Can you work these out from the model? Positions are in its coordinate system, mm. Face numbers are marked on the shaded views. A direction names the side the tool comes from. Coordinates: 2 decimals unless noted, no trailing zeros. Loops run counter-clockwise (first coordinate to the right, second up) from the corner with the lowest first, then second, coordinate; pieces in that order, holes last. Notation, with made-up numbers: (13.25, 9) -> (55.25, 9) arc R29 cw to (55.25, 31) -> close; hole circle Ø11 at (-8.5, 20.5). An arc over 180 degrees is marked (long way). Put each result on its own line as item: value. Start each with the question number.
Item 1: For the marked faces 1, 2, 3 and 4, which set-ups out of +Z, -Z, +X, -X, +Y, -Y let a thin tool reach every point of the face, with its end or its side?
Item 2: We'd pull the mould along Z, two halves only. Please class the marked faces 5, 6, 7 and 8: pulls with the +Z half, pulls with the -Z half, needs draft (parallel to the pull), parting line crosses it, or undercut.
Item 3: If we section it at A-A on z = -65.5: Please give me the cut outline in (x, y), plus the area to 3 significant figures.
Item 4: If we section it at C-C on y = 19: Please give me the cut outline in (x, z).
Item 5: If we section it at B-B on x = 30.5: Please give me the cut outline in (y, z), plus the area to 3 significant figures.
Item 6: Please list where these lines run through material, in increasing order: L1, parallel to Z at x = -146, y = 3; L2, parallel to X at y = 8.5, z = 21; L3, parallel to X at y = 27, z = -20. Write a range as from..to.
Item 7: Will these pins go through, and if not, where does the flat tip stop? P1, Ø4, axis at x = -62, z = 29, coming from the +Y side; P2, Ø1, axis at y = 29, z = -21, coming from the +X side; P3, Ø5, axis at y = 42.5, z = 27.5, coming from the -X side.
```python
from build123d import *

# Parameters (mm, degrees)
SKETCH1_W           = 300
SKETCH1_H           = 200
SKETCH1_R           = 2
BOSS_EXTRUDE1_DEPTH = 5
CUT_EXTRUDE1_REACH  = 182.347
SKETCH3_W           = 80
SKETCH3_H           = 180
SKETCH4_W           = 30
SKETCH4_H           = 60
BOSS_EXTRUDE2_DEPTH = 50
BOSS_EXTRUDE3_DEPTH = 45
SKETCH7_R           = 1.5
CUT_EXTRUDE2_DEPTH  = 5


with BuildPart() as part:
    # Sketch1 → Boss-Extrude1 (new body)
    with BuildSketch(Plane(origin=(0, 0, 0), x_dir=(1, 0, 0), z_dir=(0, 1, 0))):
        Rectangle(SKETCH1_W, SKETCH1_H)
        with Locations(Location((-146, 96, 0), (0, 0, 270))):
            Circle(SKETCH1_R, mode=Mode.SUBTRACT)
        with Locations(Location((146, 96, 0), (0, 0, 90))):
            Circle(SKETCH1_R, mode=Mode.SUBTRACT)
        with Locations(Location((146, -96, 0), (0, 0, 270))):
            Circle(SKETCH1_R, mode=Mode.SUBTRACT)
        with Locations(Location((-146, -96, 0), (0, 0, 90))):
            Circle(SKETCH1_R, mode=Mode.SUBTRACT)
    extrude(amount=BOSS_EXTRUDE1_DEPTH)

    # Sketch3 → Cut-Extrude1 (cut, up to next)
    with BuildSketch(Plane(origin=(0, 5, 0), x_dir=(1, 0, 0), z_dir=(0, 1, 0)), mode=Mode.PRIVATE) as cut_extrude1_sk1:
        Rectangle(SKETCH3_W, SKETCH3_H)
    cut_extrude1_tool1 = extrude(cut_extrude1_sk1.sketch, amount=-CUT_EXTRUDE1_REACH, mode=Mode.PRIVATE) & part.part
    add(cut_extrude1_tool1.solids().sort_by_distance((0, 5, 0))[0], mode=Mode.SUBTRACT)

    # Sketch4 → Boss-Extrude2 (add)
    with BuildSketch(Plane(origin=(0, 5, 0), x_dir=(1, 0, 0), z_dir=(0, 1, 0))):
        with Locations((-100, 0)):
            Rectangle(SKETCH4_W, SKETCH4_H)
    boss_extrude2 = extrude(amount=BOSS_EXTRUDE2_DEPTH)

    # Sketch5 → Boss-Extrude3 (add)
    with BuildSketch(Plane(origin=(-85, 0, 0), x_dir=(0, 0, -1), z_dir=(1, 0, 0))):
        with BuildLine():
            Line((-26.2, 38.191891423), (-30, 38.191891423))
            Line((-30, 38.191891423), (-30, 5))
            Line((-30, 5), (30, 5))
            Line((30, 5), (30, 38.191891423))
            Line((30, 38.191891423), (26.2, 38.191891423))
            ThreePointArc((26.2, 38.191891423), (0, 11.991891423), (-26.2, 38.191891423))
        make_face()
    boss_extrude3 = extrude(amount=BOSS_EXTRUDE3_DEPTH)

    # Sketch7 → Cut-Extrude2 (cut)
    with BuildSketch(Plane(origin=(-85, 0, 0), x_dir=(0, 0, -1), z_dir=(1, 0, 0))):
        with Locations((0, 28.765136386)):
            Circle(SKETCH7_R)
    cut_extrude2 = extrude(amount=-CUT_EXTRUDE2_DEPTH, mode=Mode.SUBTRACT)

    # Mirror3: Boss-Extrude2, Boss-Extrude3, Cut-Extrude2 across plane
    add(boss_extrude2.mirror(Plane(origin=(0, 0, 0), x_dir=(0, 0, 1), z_dir=(1, 0, 0))))
    add(boss_extrude3.mirror(Plane(origin=(0, 0, 0), x_dir=(0, 0, 1), z_dir=(1, 0, 0))))
    add(cut_extrude2.mirror(Plane(origin=(0, 0, 0), x_dir=(0, 0, 1), z_dir=(1, 0, 0))), mode=Mode.SUBTRACT)


solid = part.part
```
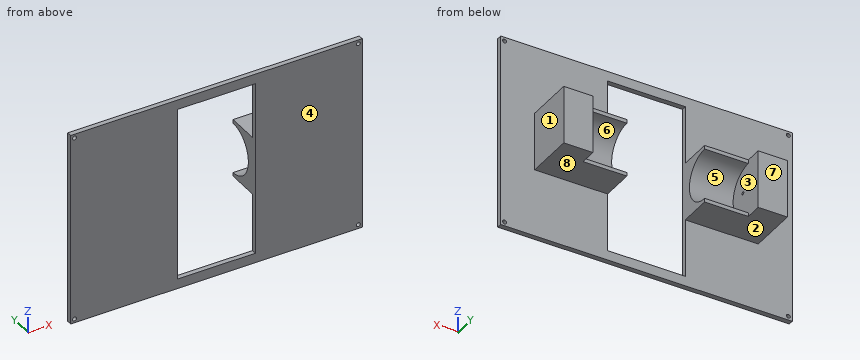
Solutions:
1. face 1: +Z, -Z, +X, +Y
1. face 2: -Z, +X, -X, +Y
1. face 3: +Y
1. face 4: +Z, -Z, +X, -X, -Y
2. face 5: undercut
2. face 6: undercut
2. face 7: needs draft
2. face 8: pulls with the -Z half
3. outline: (-150, 0) -> (-40, 0) -> (-40, 5) -> (-150, 5) -> close; (40, 0) -> (150, 0) -> (150, 5) -> (40, 5) -> close
3. area: 1,100 mm^2
4. outline: (-115, -30) -> (-40, -30) -> (-40, -17.84) -> (-85, -17.84) -> (-85, 17.84) -> (-40, 17.84) -> (-40, 30) -> (-115, 30) -> close; (40, -30) -> (115, -30) -> (115, 30) -> (40, 30) -> (40, 17.84) -> (85, 17.84) -> (85, -17.84) -> (40, -17.84) -> close
5. outline: (0, -100) -> (5, -100) -> (5, -90) -> (0, -90) -> close; (0, 90) -> (5, 90) -> (5, 100) -> (0, 100) -> close
5. area: 100 mm^2
6. L1: -100..-98, -94..94, 98..100
6. L2: -115..-40, 40..115
6. L3: -115..-85, 85..115
7. P1: y = 38.19
7. P2: x = 115
7. P3: x = -115
